Work out the finished part from the listing and answer in its coordinate system (mm). Face numbers are marked on the shaded views. A direction names the side the tool comes from. Coordinates: 2 decimals unless noted, no trailing zeros. Write each loop counter-clockwise with the first axis right and the second up, starting at its lowest first coordinate (ties: lowest second). Pieces come first, ordered by that corner, then holes. Notation, with made-up numbers: (11, 80.5) - (58, 80.5) arc R24 ccw to (58, 100.5) - close; hole circle Ø1 at (18.25, 9.5). An arc over 180 degrees is marked (long way). Use a Markdown table: item, result. Add a question column.
(1) The part is cut by section C-C, the plane x = 10. Give the vertices of the cut face in (y, z), then the cut area to 3 significant figures.
(2) For a pull along X with two mould halves and no side action, classify the marked faces 1, 2 and 3 as released by +X, released by -X, zero draft, split by the parting line, or undercut.
(3) The part is cut by section B-B, the plane z = -14. Give the vertices of the cut face in (x, y), then the cut area to 3 significant figures.
(4) The part is cut by section D-D, the plane z = -10. Give the vertices of the cut face in (x, y) (3 decimals).
(5) Find the intervals of material crossed by line 1 (Y direction, x = 0, z = 1.2); line 2 (X direction, y = -2.5, z = -18); line 3 (X direction, y = 14, z = 0.5), in increasing order. Write a range as from..to.
(6) The part is cut by section A-A, the plane y = 10.5. Give the vertices of the cut face in (x, z), then the cut area to 3 significant figures.
(7) Given pin 1 Ø5.5 at (x, z) = (-10.5, -11.5) entering from -Y; pin 2 Ø8 at (y, z) = (14.5, -6) entering from +X; pin 3 Ø2 at (y, z) = (14.5, 1) entering from -X; pin 4 Ø2 at (x, z) = (19, -11) entering from +Y, each flat-ended and moving along its own axis, determine where each tip first touches the part or whether it passes through.
(8) A tool of negligible diameter and unlimited length cuts with its end or side. For the marked faces 4, 5 and 6, from which of +Z, -Z, +X, -X, +Y, -Y can it reach the whole face along a straight path? Write none if from no direction.
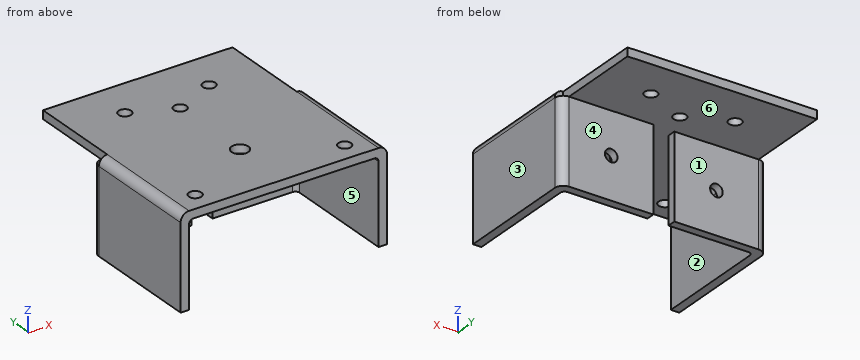
from build123d import *

# Parameters (mm, degrees)
SKETCH1_W               = 49
SKETCH1_H               = 50
BOSS_EXTRUDE1_DEPTH     = 2
SKETCH3_W               = 2
SKETCH3_H               = 22
CUT_EXTRUDE1_DEPTH      = 36.060661717
BOSS_EXTRUDE5_DEPTH     = 20
FILLET3_R               = 2
FILLET4_R               = 1
SKETCH8_R               = 2
SKETCH8_R_2             = 1.5
CUT_EXTRUDE2_DEPTH      = 10
CUT_EXTRUDE3_DEPTH      = 44.591857038
CUT_EXTRUDE3_DEPTH_BACK = 44.591857038
SKETCH9_R               = 1.5


with BuildPart() as part:
    # Sketch1 → Boss-Extrude1 (new body)
    with BuildSketch(Plane.XY):
        Rectangle(SKETCH1_W, SKETCH1_H)
    extrude(amount=BOSS_EXTRUDE1_DEPTH)

    # Sketch3 → Cut-Extrude1 (cut, through all)
    with BuildSketch(Plane.XY.offset(2)):
        with Locations((-23.5, 14)):
            Rectangle(SKETCH3_W, SKETCH3_H)
        with Locations((23.5, 14)):
            Rectangle(SKETCH3_W, SKETCH3_H)
    extrude(amount=-CUT_EXTRUDE1_DEPTH, mode=Mode.SUBTRACT)

    # Sketch7 → Boss-Extrude5 (add)
    with BuildSketch(Plane(origin=(0, 0, 0), x_dir=(-1, 0, 0), z_dir=(0, 0, -1))):
        Polygon((-24.5, -25), (-24.5, 5), (-2.49, 5), (-2.49, 3), (-22.49, 3), (-22.49, -25), align=None)
        Polygon((24.5, 5), (2.49, 5), (2.49, 3), (22.49, 3), (22.49, -25), (24.5, -25), align=None)
    extrude(amount=BOSS_EXTRUDE5_DEPTH)

    # Fillet3
    fillet3_edges = [part.edges().sort_by_distance(p)[0] for p in [
        (-24.5, 5, -10),
        (24.5, 5, -10),
        (-24.5, -11, 2),
        (24.5, -11, 2),
    ]]
    fillet(fillet3_edges, radius=FILLET3_R)

    # Fillet4
    fillet4_edges = [part.edges().sort_by_distance(p)[0] for p in [
        (22.49, -11, 0),
        (22.49, 3, -10),
        (-22.49, -11, 0),
        (-22.49, 3, -10),
    ]]
    fillet(fillet4_edges, radius=FILLET4_R)

    # Sketch8 → Cut-Extrude2 (cut)
    with BuildSketch(Plane.XY.offset(2)):
        with Locations((0, -10)):
            Circle(SKETCH8_R)
        with Locations((0, 10.5)):
            Circle(SKETCH8_R_2)
        with Locations((17.753520778, -20.25)):
            Circle(SKETCH8_R_2)
        with Locations((-17.753520778, -20.25)):
            Circle(SKETCH8_R_2)
        with Locations((-10, 15)):
            Circle(SKETCH8_R_2)
        with Locations(Location((10, 15, 0), (0, 0, 180))):
            Circle(SKETCH8_R_2)
    extrude(amount=-CUT_EXTRUDE2_DEPTH, mode=Mode.SUBTRACT)

    # Sketch9 → Cut-Extrude3 (cut, two sides: drawn at the far end of the back side and taken through both)
    with BuildSketch(Plane(origin=(0, 5, 0), x_dir=(1, 0, 0), z_dir=(0, 1, 0)).offset(-CUT_EXTRUDE3_DEPTH_BACK)):
        with Locations(Location((12.495, 10, 0), (0, 0, 270))):
            Circle(SKETCH9_R)
        with Locations(Location((-12.495, 10, 0), (0, 0, 270))):
            Circle(SKETCH9_R)
    extrude(amount=CUT_EXTRUDE3_DEPTH + CUT_EXTRUDE3_DEPTH_BACK, mode=Mode.SUBTRACT)


solid = part.part
Model answer:
| question | item | result |
|---|---|---|
| 1 | outline | (-25, 0) - (3, 0) - (3, -20) - (5, -20) - (5, 0) - (13.5, 0) - (13.5, 2) - (-25, 2) - close; (16.5, 0) - (25, 0) - (25, 2) - (16.5, 2) - close |
| 1 | area | 134 mm^2 |
| 2 | face 1 | zero draft |
| 2 | face 2 | undercut |
| 2 | face 3 | released by +X |
| 3 | outline | (-24.5, -25) - (-22.49, -25) - (-22.49, 2) arc R1 cw to (-21.49, 3) - (-2.49, 3) - (-2.49, 5) - (-22.5, 5) arc R2 ccw to (-24.5, 3) - close; (2.49, 3) - (21.49, 3) arc R1 cw to (22.49, 2) - (22.49, -25) - (24.5, -25) - (24.5, 3) arc R2 ccw to (22.5, 5) - (2.49, 5) - close |
| 3 | area | 199 mm^2 |
| 4 | outline | (-24.5, -25) - (-22.49, -25) - (-22.49, 2) arc R1 cw to (-21.49, 3) - (-13.995, 3) - (-13.995, 5) - (-22.5, 5) arc R2 ccw to (-24.5, 3) - close; (-10.995, 3) - (-2.49, 3) - (-2.49, 5) - (-10.995, 5) - close; (2.49, 3) - (10.995, 3) - (10.995, 5) - (2.49, 5) - close; (13.995, 3) - (21.49, 3) arc R1 cw to (22.49, 2) - (22.49, -25) - (24.5, -25) - (24.5, 3) arc R2 ccw to (22.5, 5) - (13.995, 5) - close |
| 5 | line 1 | -25..-12, -8..9, 12..25 |
| 5 | line 2 | -24.5..-22.49, 22.49..24.5 |
| 5 | line 3 | -22.5..-11.12, -8.88..8.88, 11.12..22.5 |
| 6 | outline | (-22.5, 0) - (-1.5, 0) - (-1.5, 2) - (-22.5, 2) - close; (1.5, 0) - (22.5, 0) - (22.5, 2) - (1.5, 2) - close |
| 6 | area | 84.0 mm^2 |
| 7 | pin 1 | y = 3 |
| 7 | pin 2 | through |
| 7 | pin 3 | x = -22.5 |
| 7 | pin 4 | y = 5 |
| 8 | face 4 | -Z, +X, -X, +Y |
| 8 | face 5 | -Z, -Y |
| 8 | face 6 | -Z |
